Model file for the job. Use its own axes, mm. Round coordinates to 2 decimals unless told otherwise and drop trailing zeros. Order: outer loops, then holes, each group sorted by start corner. A loop starts at its lowest first (then second) coordinate and runs counter-clockwise, first axis right, second up. Notation, with made-up numbers: (67.5, 17.25) -> (126.5, 17.25) arc R12 cw to (126.5, 35.25) -> close; hole circle Ø3 at (58, 22). An arc over 180 degrees is marked (long way). Use CSV: the item, a comma, the result in double quotes.
```python
from build123d import *

# Parameters (mm, degrees)
SKETCH1_W           = 609.6
SKETCH1_H           = 279.4
BOSS_EXTRUDE1_DEPTH = 3.175
SKETCH1_9_R         = 3.822247212
SKETCH1_9_R_2       = 3.81
CUT_EXTRUDE1_DEPTH  = 414.49423288
SKETCH1_10_R        = 3.822247212
SKETCH1_10_R_2      = 3.81
CUT_EXTRUDE2_DEPTH  = 414.49423288


with BuildPart() as part:
    # Sketch1 → Boss-Extrude1 (new body)
    with BuildSketch(Plane.XY):
        with Locations((0, -139.7)):
            Rectangle(SKETCH1_W, SKETCH1_H)
    extrude(amount=-BOSS_EXTRUDE1_DEPTH)

    # Sketch1_9 → Cut-Extrude1 (cut, through all)
    with BuildSketch(Plane.XY):
        Polygon((-135.382, -19.05), (-174.272872965, -57.940872965), (-151.291902577, -80.921843354), (-112.401029611, -42.030970389), align=None)
        Polygon((-225.973143095, -139.849843354), (-187.08227013, -178.740716319), (-164.101299742, -155.759745931), (-202.992172707, -116.868872965), align=None)
        Polygon((174.272872965, -57.940872965), (151.291902577, -80.921843354), (112.401029611, -42.030970389), (135.382, -19.05), align=None)
        Polygon((187.08227013, -178.740716319), (164.101299742, -155.759745931), (202.992172707, -116.868872965), (225.973143095, -139.849843354), align=None)
        with Locations((-131.038243043, -75.755014104)):
            Circle(SKETCH1_9_R)
        with Locations(Location((-100.325767109, -106.467490038, 0), (0, 0, 180))):
            Circle(SKETCH1_9_R)
        with Locations((-238.048405598, -204.286363003)):
            Circle(SKETCH1_9_R_2)
        with Locations(Location((-207.335929664, -173.573887069, 0), (0, 0, 180))):
            Circle(SKETCH1_9_R_2)
        with Locations(Location((-117.567858862, -62.284629922, 0), (0, 0, 180))):
            Circle(SKETCH1_9_R)
        with Locations((-86.855382928, -92.997105856)):
            Circle(SKETCH1_9_R)
        with Locations((-220.806313845, -160.103502887)):
            Circle(SKETCH1_9_R_2)
        with Locations(Location((-251.518789779, -190.815978821, 0), (0, 0, 180))):
            Circle(SKETCH1_9_R_2)
    extrude(amount=-CUT_EXTRUDE1_DEPTH, mode=Mode.SUBTRACT)

    # Sketch1_10 → Cut-Extrude2 (cut, through all)
    with BuildSketch(Plane.XY):
        with Locations((131.038243043, -75.755014104)):
            Circle(SKETCH1_10_R)
        with Locations((117.567858862, -62.284629922)):
            Circle(SKETCH1_10_R)
        with Locations((86.855382928, -92.997105856)):
            Circle(SKETCH1_10_R)
        with Locations((100.325767109, -106.467490038)):
            Circle(SKETCH1_10_R)
        with Locations((238.048405598, -204.286363003)):
            Circle(SKETCH1_10_R_2)
        with Locations((251.518789779, -190.815978821)):
            Circle(SKETCH1_10_R_2)
        with Locations((220.806313845, -160.103502887)):
            Circle(SKETCH1_10_R_2)
        with Locations((207.335929664, -173.573887069)):
            Circle(SKETCH1_10_R_2)
    extrude(amount=-CUT_EXTRUDE2_DEPTH, mode=Mode.SUBTRACT)


solid = part.part
```
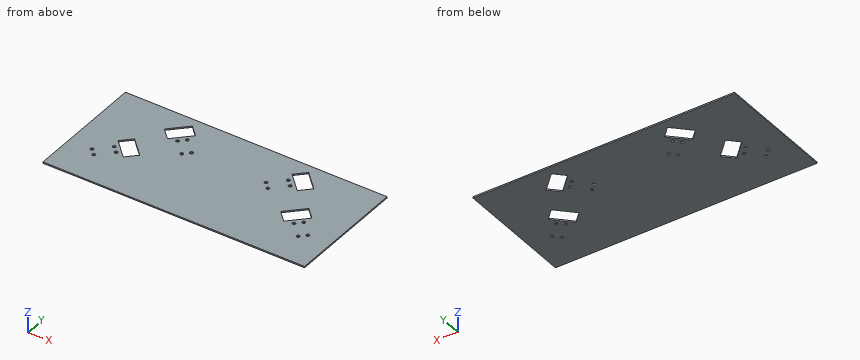
Q1. Probe line 1 along X through (y, z) = (-48.5, -1.4); line 2 along X through (y, z) = (-104, -2.95); line 3 along X through (y, z) = (-72.5, -0.5). List the from-to ranges inside material, lowest first.
From the geometry:
line 1,"x = -304.8 to -164.83, -118.87 to 118.87, 164.83 to 304.8"
line 2,"x = -304.8 to -103.24, -97.41 to 97.41, 103.24 to 304.8"
line 3,"x = -304.8 to -159.71, -142.87 to -133.04, -129.03 to 129.03, 133.04 to 142.87, 159.71 to 304.8"
Q2. Cut at A-A (y = -124). Give the cut face in (x, z) (3 decimals), plus the area to 3 significant figures.
From the geometry:
outline,"(-304.8, -3.175) -> (-210.123, -3.175) -> (-210.123, 0) -> (-304.8, 0) -> close; (-195.861, -3.175) -> (195.861, -3.175) -> (195.861, 0) -> (-195.861, 0) -> close; (210.123, -3.175) -> (304.8, -3.175) -> (304.8, 0) -> (210.123, 0) -> close"
area,"1,840 mm²"
Q3. Cut at B-B (z = -1.9). State how many separate pieces and enclosed holes the cut face has, plus the area to 3 significant figures.
From the geometry:
separate pieces,"1"
enclosed holes,"20"
area,"162,000 mm²"
